from build123d import *

# Parameters (mm, degrees)
SKETCH3_R = 0.1651
FILLET1_R = 0.1651


with BuildPart() as part:
    # Sweep1: sweep along a path in Sketch2
    with BuildLine(Plane.XY) as sweep1_path:
        Line((16.5989, -2.0066), (16.5989, -3.4925))
        ThreePointArc((16.5989, -3.4925), (15.434620166, -6.303320166), (12.6238, -7.4676))
        Line((12.6238, -7.4676), (-12.6238, -7.4676))
        ThreePointArc((-12.6238, -7.4676), (-15.434620166, -6.303320166), (-16.5989, -3.4925))
        Line((-16.5989, -3.4925), (-16.5989, 4.2926))
    # Sketch3 → Sweep1 (sweep)
    with BuildSketch(Plane(origin=(0, 4.2926, 0), x_dir=(-1, 0, 0), z_dir=(0, 1, 0))):
        with Locations((16.4338, 0)):
            Circle(SKETCH3_R)
    sweep(path=sweep1_path.line)

    # Fillet1
    fillet1_edges = [part.edges().sort_by_distance(p)[0] for p in [
        (16.2687, -2.0066, 0),
    ]]
    fillet(fillet1_edges, radius=FILLET1_R)


solid = part.part
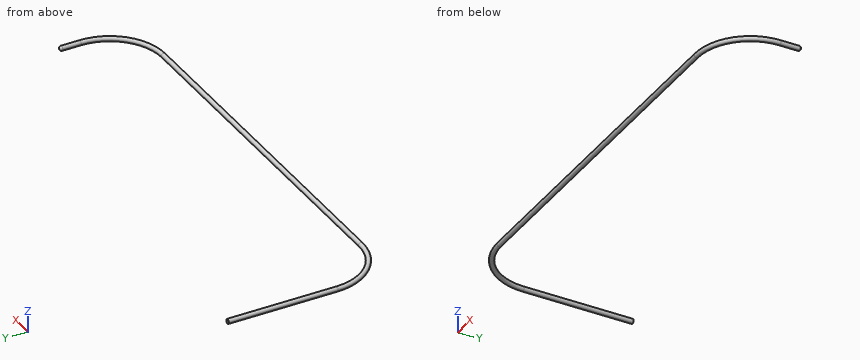
For this review, take the finished solid that the model builds, in its own axes (mm). Give positions to 0.01 mm unless a question says otherwise; leave off trailing zeros. Order: outer loops, then holes, each group sorted by start corner. A loop starts at its lowest first (then second) coordinate and runs counter-clockwise, first axis right, second up. Notation, with made-up numbers: M 43.25,66.25 L 72.25,66.25 A17 cw 72.25,88.25 Z; hole C 20,-10.75 d4. An arc over 180 degrees is marked long. Answer in a Markdown table with one row per item. Add a question column.
(1) For pin 1 (5 mm diameter, centred on x = 9, y = -3, fed in from -Z), flat-tipped, find the tip position at first contact; note if it passes through.
(2) Consider section D-D on y = 1.75. State the section outline as (x, z) points.
(3) Consider section A-A on z = 0. State the section outline as (x, y) points.
(4) Consider section B-B on y = -2.5. State the section outline as (x, z) points, and give its area (3 significant figures).
(5) Wall thickness on probe 1 along Y at (x, z) = (6, 0.05); probe 2 along X at (y, z) = (-6.5, -0.05); probe 3 along Y at (x, z) = (-8, -0.1): over which ranges is each line inside the solid? List them lowest first. Write a range as [from, to].
(6) Consider section C-C on x = 9. State the section outline as (y, z) points, and give its area (3 significant figures).
Evaluation:
| question | item | result |
|---|---|---|
| 1 | pin 1 | passes through |
| 2 | outline | C -16.43,0 d0.33 |
| 3 | outline | M -16.6,-3.49 A3.98 ccw -12.62,-7.47 L 12.62,-7.47 A3.98 ccw 16.6,-3.49 L 16.6,-2.17 A0.17 ccw 16.27,-2.17 L 16.27,-3.49 A3.64 cw 12.62,-7.14 L -12.62,-7.14 A3.64 cw -16.27,-3.49 L -16.27,4.29 L -16.6,4.29 Z |
| 4 | outline | C -16.43,0 d0.33; C 16.43,0 d0.33 |
| 4 | area | 0.171 mm^2 |
| 5 | probe 1 | y = [-7.46, -7.15] |
| 5 | probe 2 | x = [-15.21, -14.7], [14.7, 15.21] |
| 5 | probe 3 | y = [-7.43, -7.17] |
| 6 | outline | C -7.3,0 d0.33 |
| 6 | area | 0.0856 mm^2 |
